The model under review builds one solid part; all positions refer to its coordinate system, in mm. Face numbers are marked on the shaded views. A direction names the side the tool comes from. Coordinates: 2 decimals unless noted, no trailing zeros. Loops run counter-clockwise (first coordinate to the right, second up) from the corner with the lowest first, then second, coordinate; pieces in that order, holes last. Notation, with made-up numbers: M -9.75,-13.5 L 10.25,-13.5 A18 cw 10.25,6.5 Z; hole C -27.75,69.5 d8. An arc over 180 degrees is marked long. Return JSON: item names as keys, results as strings.
```python
from build123d import *

# Parameters (mm, degrees)
SKIZZE1_W                       = 300
SKIZZE1_H                       = 57
SKIZZE1_R                       = 2.1
BASIS_BLECH1_DEPTH              = 2
KANTE_LASCHE1_STRIP_W           = 8.2
KANTE_LASCHE1_STRIP_H           = 2
KANTE_LASCHE1_STRIP_CUT_DEPTH   = 57
KANTE_LASCHE1_STRIP_2_W         = 8.2
KANTE_LASCHE1_STRIP_2_H         = 2
KANTE_LASCHE1_STRIP_CUT_2_DEPTH = 57
KANTE_LASCHE1_DEPTH             = 57
KANTE_LASCHE1_BEND_DEPTH        = 57
SKIZZE10_R                      = 2.1
SCHNITT_LINEAR_AUSTRAGEN1_DEPTH = 381.921579856


# Sheet-metal steps are written as plain solids
with BuildPart() as part:
    # Skizze1 → Basis-Blech1 (new body)
    with BuildSketch(Plane.XY):
        Rectangle(SKIZZE1_W, SKIZZE1_H)
        with Locations((-117, 6)):
            Circle(SKIZZE1_R, mode=Mode.SUBTRACT)
        with Locations((117, 6)):
            Circle(SKIZZE1_R, mode=Mode.SUBTRACT)
    extrude(amount=-BASIS_BLECH1_DEPTH)

    # Kante-Lasche1 strip (across the edge) → Kante-Lasche1 strip cut (cut)
    with BuildSketch(Plane(origin=(-150, 28.5, 0), x_dir=(1, 0, 0), z_dir=(0, -1, 0))):
        with Locations((-2, -1)):
            Rectangle(KANTE_LASCHE1_STRIP_W, KANTE_LASCHE1_STRIP_H)
    extrude(amount=KANTE_LASCHE1_STRIP_CUT_DEPTH, mode=Mode.SUBTRACT)

    # Kante-Lasche1 strip 2 (across the edge) → Kante-Lasche1 strip cut 2 (cut)
    with BuildSketch(Plane(origin=(150, -28.5, 0), x_dir=(-1, 0, 0), z_dir=(0, 1, 0))):
        with Locations((-2, -1)):
            Rectangle(KANTE_LASCHE1_STRIP_2_W, KANTE_LASCHE1_STRIP_2_H)
    extrude(amount=KANTE_LASCHE1_STRIP_CUT_2_DEPTH, mode=Mode.SUBTRACT)

    # Kante-Lasche1 section (across the edge) → Kante-Lasche1 (add)
    with BuildSketch(Plane(origin=(-150, 28.5, 0), x_dir=(1, 0, 0), z_dir=(0, -1, 0))):
        with BuildLine():
            Line((0, 0.1), (0, 233))
            Line((0, 233), (2, 233))
            Line((2, 233), (2, 0.1))
            ThreePointArc((2, 0.1), (2.029289322, 0.029289322), (2.1, 0))
            Line((2.1, 0), (2.1, -2))
            ThreePointArc((2.1, -2), (0.61507576, -1.38492424), (0, 0.1))
        make_face()
    extrude(amount=KANTE_LASCHE1_DEPTH)

    # Kante-Lasche1 section 2 (across the edge) → Kante-Lasche1 bend (add)
    with BuildSketch(Plane(origin=(150, -28.5, 0), x_dir=(-1, 0, 0), z_dir=(0, 1, 0))):
        with BuildLine():
            Line((0, 0.1), (0, 233))
            Line((0, 233), (2, 233))
            Line((2, 233), (2, 0.1))
            ThreePointArc((2, 0.1), (2.029289322, 0.029289322), (2.1, 0))
            Line((2.1, 0), (2.1, -2))
            ThreePointArc((2.1, -2), (0.61507576, -1.38492424), (0, 0.1))
        make_face()
    extrude(amount=KANTE_LASCHE1_BEND_DEPTH)

    # Skizze10 → Schnitt-Linear austragen1 (cut, through all)
    with BuildSketch(Plane(origin=(150, 0, 0), x_dir=(0, 0, -1), z_dir=(1, 0, 0))):
        with Locations((-191, 6)):
            Circle(SKIZZE10_R)
    extrude(amount=-SCHNITT_LINEAR_AUSTRAGEN1_DEPTH, mode=Mode.SUBTRACT)


solid = part.part
```
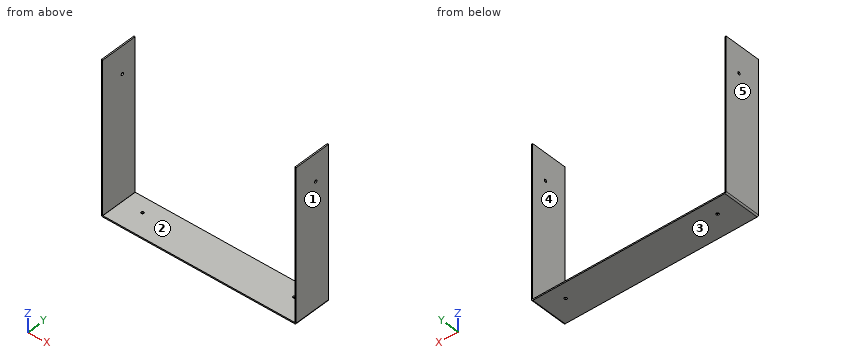
1. Machinability: for the marked faces 1 and 2, which of the approach directions +Z, -Z, +X, -X, +Y, -Y give a long, thin tool a straight path to every point of the face, cutting with its end or side? Answer none if there is none.
Check values:
{"face 1": "+Z, -Z, +X, +Y, -Y", "face 2": "+Z, +Y, -Y"}
2. The part is to be moulded in two halves that separate along X. For the marked faces 3, 4 and 5, say which applies: released by +X, released by -X, zero draft, split by the parting line, or undercut.
Check values:
{"face 3": "zero draft", "face 4": "undercut", "face 5": "released by -X"}
3. Add section C-C on x = 9.5. Give the boundary of the cut face in (y, z).
Check values:
{"outline": "M -28.5,-2 L 28.5,-2 L 28.5,0 L -28.5,0 Z"}
4. Insertion check: pin 1 Ø12 at (x, y) = (75.5, 9.5) entering from +Z; pin 2 Ø3.5 at (y, z) = (6, 191) entering from +X. Each pin has a flat end and moves straight along its axis. Give the tip position at first contact, or say it passes through.
Check values:
{"pin 1": "z = 0", "pin 2": "through"}
5. Add section B-B on y = 17.5. Give the boundary of the cut face in (x, z).
Check values:
{"outline": "M -150,0.1 A2.1 ccw -147.9,-2 L 147.9,-2 A2.1 ccw 150,0.1 L 150,233 L 148,233 L 148,0.1 A0.1 cw 147.9,0 L -147.9,0 A0.1 cw -148,0.1 L -148,233 L -150,233 Z"}
6. Add section A-A on z = 104. Give the boundary of the cut face in (x, y), plus the area to 3 significant figures.
Check values:
{"outline": "M -150,-28.5 L -148,-28.5 L -148,28.5 L -150,28.5 Z; M 148,-28.5 L 150,-28.5 L 150,28.5 L 148,28.5 Z", "area": "228 mm²"}
7. To check wall thickness, follow line 1 (X direction, y = 21, z = 122); line 2 (Y direction, x = 149, z = 191); line 3 (Z direction, x = 55.5, y = 15.5). State the ranges of each line that lie inside material, in increasing order.
Check values:
{"line 1": "-150 to -148, 148 to 150", "line 2": "-28.5 to 3.9, 8.1 to 28.5", "line 3": "-2 to 0"}
